```python
from build123d import *

# Parameters (mm, degrees)
SKETCH1_W           = 25
SKETCH1_H           = 25
BOSS_EXTRUDE1_DEPTH = 37
SKETCH2_W           = 30.6
SKETCH2_H           = 19
CUT_EXTRUDE1_DEPTH  = 22
SKETCH3_W           = 25
SKETCH3_H           = 25
CUT_EXTRUDE2_DEPTH  = 3
SKETCH4_W           = 6
SKETCH4_H           = 25
BOSS_EXTRUDE2_DEPTH = 5
BOSS_EXTRUDE3_DEPTH = 0.8
BOSS_EXTRUDE4_DEPTH = 0.8


with BuildPart() as part:
    # Sketch1 → Boss-Extrude1 (new body)
    with BuildSketch(Plane(origin=(0, 0, 0), x_dir=(0, 0, -1), z_dir=(1, 0, 0))):
        with Locations((12.5, -12.5)):
            Rectangle(SKETCH1_W, SKETCH1_H)
    extrude(amount=BOSS_EXTRUDE1_DEPTH)

    # Sketch2 → Cut-Extrude1 (cut)
    with BuildSketch(Plane.XZ.offset(25)):
        with Locations((18.5, -9.5)):
            Rectangle(SKETCH2_W, SKETCH2_H)
    extrude(amount=-CUT_EXTRUDE1_DEPTH, mode=Mode.SUBTRACT)

    # Sketch3 → Cut-Extrude2 (cut)
    with BuildSketch(Plane(origin=(0, 0, -25), x_dir=(-1, 0, 0), z_dir=(0, 0, -1))):
        with Locations((-18.5, -12.5)):
            Rectangle(SKETCH3_W, SKETCH3_H)
    extrude(amount=-CUT_EXTRUDE2_DEPTH, mode=Mode.SUBTRACT)

    # Sketch4 → Boss-Extrude2 (add)
    with BuildSketch(Plane(origin=(0, 0, -25), x_dir=(-1, 0, 0), z_dir=(0, 0, -1))):
        with Locations((-34, -12.5)):
            Rectangle(SKETCH4_W, SKETCH4_H)
        with Locations((-3, -12.5)):
            Rectangle(SKETCH4_W, SKETCH4_H)
    extrude(amount=BOSS_EXTRUDE2_DEPTH)

    # Sketch5 → Boss-Extrude3 (add)
    with BuildSketch(Plane(origin=(6, 0, 0), x_dir=(0, 0, -1), z_dir=(1, 0, 0))):
        Polygon((30, -15), (27.633974643, -15), (28.5, -23.5), (27.394305398, -23.5), (26.528280041, -15), (22, -15), (22, -25), (30, -25), align=None)
    extrude(amount=BOSS_EXTRUDE3_DEPTH)

    # Sketch6 → Boss-Extrude4 (add)
    with BuildSketch(Plane.ZY.offset(-31)):
        Polygon((-30, -15), (-30, -25), (-22, -25), (-22, -15), (-26.528280041, -15), (-27.394305398, -23.5), (-28.5, -23.5), (-27.633974643, -15), align=None)
    extrude(amount=BOSS_EXTRUDE4_DEPTH)


solid = part.part
```
Could you check a few things on this model? Use its own coordinates, in mm. A direction names the side the tool comes from. Give positions to 0.01 mm unless a question says otherwise; leave off trailing zeros. Write each loop counter-clockwise with the first axis right and the second up, starting at its lowest first coordinate (ties: lowest second). Pieces come first, ordered by that corner, then holes. Notation, with made-up numbers: (-27.75, 37) -> (-17.75, 37) arc R18 cw to (-17.75, 57) -> close; hole circle Ø6 at (37.5, -35). An arc over 180 degrees is marked (long way). Write each question's results on one line, items separated by ' | '.
1. I want a section at B-B, the plane y = -7. Write out the boundary of the cut face in (x, z).
Check sheet entries:
outline: (0, -30) -> (6, -30) -> (6, -22) -> (31, -22) -> (31, -30) -> (37, -30) -> (37, 0) -> (33.8, 0) -> (33.8, -19) -> (3.2, -19) -> (3.2, 0) -> (0, 0) -> close
2. I want a section at D-D, the plane z = -6.5. Write out the boundary of the cut face in (x, y), then the cut area to 3 significant figures.
Check sheet entries:
outline: (0, -25) -> (3.2, -25) -> (3.2, -3) -> (33.8, -3) -> (33.8, -25) -> (37, -25) -> (37, 0) -> (0, 0) -> close | area: 252 mm²
3. On a 3-axis mill with a long thin cutter (end or side, diameter ignored), from which of +Z, -Z, +X, -X, +Y, -Y can I reach the whole of each face in a straight line? I mean faces 5 (the flat face through (18, -14, -19)), 6 (the flat face through (6.39, -19.19, -28.06)), 7 (the flat face through (30.606, -19.19, -26.955)), 8 (the flat face through (0, -12, -15)), 9 (the flat face through (6.8, -20, -26)). Say none if no direction works.
Check sheet entries:
face 5: +Z, -Y | face 6: none | face 7: +Y | face 8: +Z, -Z, -X, +Y, -Y | face 9: -Z, +Y, -Y
4. If we mould it in two halves opening along X, with no side actions, what happens to faces 1 (the flat face through (6.394, -19.31, -26.967)), 2 (the flat face through (30.606, -19.31, -28.073)), 3 (the flat face through (37, -13, -15)), 4 (the flat face through (19, -25, -20))? For each: released by +X, released by -X, zero draft, split by the parting line, or undercut.
Check sheet entries:
face 1: undercut | face 2: undercut | face 3: released by +X | face 4: zero draft
5. I want a section at C-C, the plane x = 33. Write out the boundary of the cut face in (y, z), then the cut area to 3 significant figures.
Check sheet entries:
outline: (-25, -30) -> (0, -30) -> (0, 0) -> (-3, 0) -> (-3, -19) -> (-25, -19) -> close | area: 332 mm²
6. Will these pins go through, and if not, where does the flat tip stop? pin 1 Ø0.9 at (x, z) = (30.5, -29) entering from +Y; pin 2 Ø7.5 at (x, y) = (14, -10.5) entering from -Z; pin 3 Ø12 at (x, y) = (13, -16.5) entering from +Z.
Check sheet entries:
pin 1: stops at y = -15 | pin 2: stops at z = -22 | pin 3: stops at z = -19
7. I want a section at A-A, the plane z = -26. Write out the boundary of the cut face in (x, y).
Check sheet entries:
outline: (0, -25) -> (6.8, -25) -> (6.8, -15) -> (6, -15) -> (6, 0) -> (0, 0) -> close; (30.2, -25) -> (37, -25) -> (37, 0) -> (31, 0) -> (31, -15) -> (30.2, -15) -> close
8. I need wall thicknesses on L1, parallel to X at y = -10.75, z = -3.25; L2, parallel to X at y = -17, z = -27.75; L3, parallel to Z at x = 16.5, y = -15.75. Which ranges of each line are inside material? Lowest first, please.
Check sheet entries:
L1: x = 0 to 3.2, 33.8 to 37 | L2: x = 0 to 6, 31 to 37 | L3: z = -22 to -19
